from build123d import *

# Parameters (mm, degrees)
F0_W     = 60
F0_H     = 30
F1_DEPTH = 30
F2_W     = 27.9342501611
F2_H     = 30
F3_DEPTH = 40
F3_TAPER = 7
F4_R     = 5
F5_DEPTH = 30


with BuildPart() as f1:
    # F0 (on Front) → F1 (new body)
    with BuildSketch(Plane.XZ):
        with Locations((-2.0657498389, 1.2521591907)):
            Rectangle(F0_W, F0_H)
    extrude(amount=F1_DEPTH)

    # F2 (on face) → F3 (join)
    with BuildSketch(Plane.XY.offset(16.2521591907)):
        with Locations((13.9671250805, -15)):
            Rectangle(F2_W, F2_H)
    extrude(amount=F3_DEPTH, taper=F3_TAPER)

    # F4 (on face) → F5 (cut)
    with BuildSketch(Plane.XY.offset(56.2521591907)):
        with Locations((14.8219978437, -14.2463846132)):
            Circle(F4_R)
    extrude(amount=-F5_DEPTH, mode=Mode.SUBTRACT)


solid = f1.part
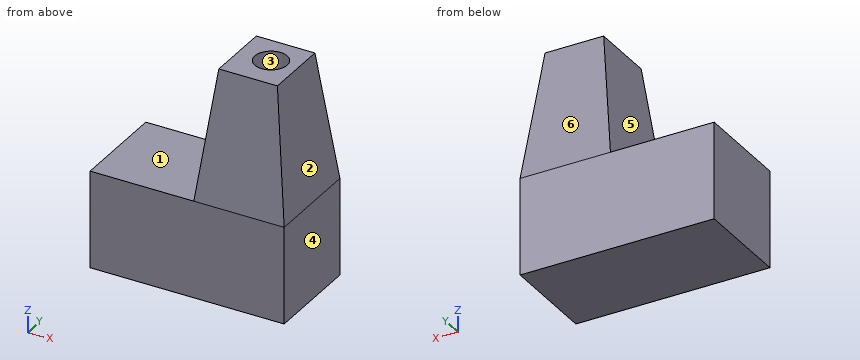
Geometry: final body of the model. Coordinates: model frame, mm. Face numbers are marked on the shaded views. A direction names the side the tool comes from. Give positions to 0.01 mm unless a question says otherwise; leave off trailing zeros. Loops run counter-clockwise (first coordinate to the right, second up) from the corner with the lowest first, then second, coordinate; pieces in that order, holes last. Notation, with made-up numbers: (-10, 4.25) - (9, 4.25) arc R10 cw to (9, 18.25) - close; hole circle Ø9 at (-17.5, -37.5). An arc over 180 degrees is marked (long way). Answer as CSV lines item,"result". Start each with the question number.
1. Section C-C, the plane z = 38. Return loops of the section in (x, y), plus the area to 3 significant figures.
2. Section A-A, the plane y = -20.5. Return loops of the section in (x, z).
3. Section B-B, the plane x = 6. Return loops of the section in (y, z), plus the area to 3 significant figures.
4. Pin query (flat end, axial travel): P1, Ø5, axis at x = 13.5, y = -14.5, coming from the +Z side; P2, Ø2, axis at y = -23.5, z = 48, coming from the -X side; P3, Ø1, axis at y = -15.5, z = 30, coming from the +X side. Return the tip coordinate at first contact, or that it passes through.
5. Draft query along X for the marked faces 3, 4, 5 and 6. Return one class per face: released by +X, released by -X, zero draft, split by the parting line, or undercut.
6. Section D-D, the plane y = -16. Return loops of the section in (x, z), plus the area to 3 significant figures.
7. Reachability of the marked faces 1 and 2 from +Z, -Z, +X, -X, +Y, -Y: full face, straight path, thin tool, end or side. Return the list, or none.
8. Ray query, L1, parallel to Z at x = -16, y = -25; L2, parallel to X at y = -15.75, z = 27; L3, parallel to X at y = -11, z = 34. Return the intervals inside material, ascending.
Answers:
1,outline,"(2.67, -27.33) - (25.26, -27.33) - (25.26, -2.67) - (2.67, -2.67) - close; hole circle Ø10 at (14.82, -14.25)"
1,area,"479 mm2"
2,outline,"(-32.07, -13.75) - (27.93, -13.75) - (27.93, 16.25) - (23.02, 56.25) - (4.91, 56.25) - (0, 16.25) - (-32.07, 16.25) - close"
3,outline,"(-30, -13.75) - (0, -13.75) - (0, 16.25) - (-4.91, 56.25) - (-25.09, 56.25) - (-30, 16.25) - close"
3,area,"1,900 mm2"
4,P1,"stops at z = 26.25"
4,P2,"stops at x = 3.78"
4,P3,"stops at x = 26.31"
5,face 3,"undercut"
5,face 4,"released by +X"
5,face 5,"released by -X"
5,face 6,"zero draft"
6,outline,"(-32.07, -13.75) - (27.93, -13.75) - (27.93, 16.25) - (23.02, 56.25) - (19.5, 56.25) - (19.5, 26.25) - (10.14, 26.25) - (10.14, 56.25) - (4.91, 56.25) - (0, 16.25) - (-32.07, 16.25) - close"
6,area,"2,440 mm2"
7,face 1,"+Z, -X, +Y, -Y"
7,face 2,"+Z, +X, +Y, -Y"
8,L1,"z = -13.75 to 16.25"
8,L2,"x = 1.32 to 10.05, 19.59 to 26.61"
8,L3,"x = 2.18 to 11.02, 18.62 to 25.76"
